Can you work these out from the model? Positions are in its coordinate system, mm. A direction names the side the tool comes from. Coordinates: 2 decimals unless noted, no trailing zeros. Loops run counter-clockwise (first coordinate to the right, second up) from the corner with the lowest first, then second, coordinate; pieces in that order, holes last.
Autodesk Inventor part; units mm, degrees
ref_plane "YZ Plane" through (0, 0, 0) normal (1, 0, 0) x (0, 1, 0)
ref_plane "XZ Plane" through (0, 0, 0) normal (0, 1, 0) x (-1, 0, 0)
ref_plane "XY Plane" through (0, 0, 0) normal (0, 0, 1) x (1, 0, 0)
sketch "Sketch1" plane through (0, 0, 0) normal (1, 0, 0) x (0, 1, 0)
  line L0 (-25.4, -50.8) -> (25.4, -50.8)
  line L1 (25.4, -50.8) -> (25.4, 50.8)
  line L2 (25.4, 50.8) -> (-25.4, 50.8)
  line L3 (-25.4, 50.8) -> (25.4, -50.8) construction
  line L4 (-25.4, -50.8) -> (25.4, 50.8) construction
  arc A0 (-25.4, -25.654) -> (-25.4, 25.654) centre (-25.4, 0) ccw
  line L5 (-25.4, 50.8) -> (-25.4, 25.654)
  line L6 (-25.4, -25.654) -> (-25.4, -50.8)
  point P0 (0, 0)
  dimension "d0" = 101.6
  dimension "d1" = 50.8
  dimension "d2" = 51.308
  dimension "d6" = 50.8
  dimension "d7" = 50.8
extrude "Extrusion1" add sketch "Sketch1" along normal mid plane 12.7
sketch "Sketch3" plane through (6.35, 0, 0) normal (1, 0, 0) x (0, 0, -1)
  circle A0 centre (0, -25.4) radius 31.75 construction
  point P0 (0, 0)
  point P1 (0, 6.35)
  point P2 (0, 6.35)
  point P3 (-27.4963, -9.525)
  point P4 (-27.4963, -41.275)
  point P5 (0, -57.15)
  point P6 (27.4963, -41.275)
  point P7 (27.4963, -9.525)
  dimension "d17" = 360
hole "Hole2" at (6.35, 6.35, 0) at (6.35, -9.525, 27.4963) at (6.35, -41.275, 27.4963) at (6.35, -57.15, 0) at (6.35, -41.275, -27.4963) at (6.35, -9.525, -27.4963) direction (-1, 0, 0) diameter 3.81 end through all
sketch "Sketch4" plane through (-6.35, 25.4, 50.8) normal (0, 1, 0) x (1, 0, 0)
  line L0 (12.7, 0) -> (0, 0) construction
  line L1 (6.35, 0) -> (6.35, 101.6) construction
  line L2 (12.7, 101.6) -> (0, 101.6) construction
  point P0 (6.35, 50.8)
  point P1 (6.35, 12.7)
  point P2 (6.35, 88.9)
  dimension "d26" = 12.7
  dimension "d27" = 12.7
hole "Hole3" at (0, 25.4, 38.1) at (0, 25.4, -38.1) direction (0, -1, 0) diameter 6.7564 end through all
sketch "Sketch5" plane through (-6.35, 25.4, 50.8) normal (0, 1, 0) x (1, 0, 0)
  circle A0 centre (6.35, 88.9) radius 3.3782
  circle A1 centre (6.35, 88.9) radius 4.0132
  circle A2 centre (6.35, 12.7) radius 3.3782
  circle A3 centre (6.35, 12.7) radius 4.0132
  point P0 (6.35, 50.8)
  dimension "d35" = 8.0264
extrude "Extrusion2" cut sketch "Sketch5" against normal blind 12.7
properties part number "BottomOfSupportForAxel" material "PBT Plastic"
(1) I want a section at A-A on y = 6.35. Write out the boundary of the cut face in (x, z) (3 decimals), then the cut area to 3 significant figures.
Check values:
outline: (-6.35, -50.8) - (6.35, -50.8) - (6.35, -1.905) - (-6.35, -1.905) - close; (-6.35, 1.905) - (6.35, 1.905) - (6.35, 50.8) - (-6.35, 50.8) - close; hole circle Ø6.756 at (0, -38.1); hole circle Ø6.756 at (0, 38.1)
area: 1,170 mm2
(2) I want a section at C-C on x = 0. Write out the boundary of the cut face in (y, z) (3 decimals), then the cut area to 3 significant figures.
Check values:
outline: (-25.4, -50.8) - (25.4, -50.8) - (25.4, -42.113) - (12.7, -42.113) - (12.7, -41.478) - (-25.4, -41.478) - close; (-25.4, -34.722) - (12.7, -34.722) - (12.7, -34.087) - (25.4, -34.087) - (25.4, 34.087) - (12.7, 34.087) - (12.7, 34.722) - (-25.4, 34.722) - (-25.4, 25.654) arc R25.654 cw to (-25.4, -25.654) - close; (-25.4, 41.478) - (12.7, 41.478) - (12.7, 42.113) - (25.4, 42.113) - (25.4, 50.8) - (-25.4, 50.8) - close; hole circle Ø3.81 at (-9.525, -27.496); hole circle Ø3.81 at (-9.525, 27.496); hole circle Ø3.81 at (6.35, 0)
area: 3,370 mm2
(3) If we mould it in two halves opening along X, with no side actions, what happens to faces 3 (the cylindrical face through (-0.149, -6.617, -41.475)), 4 (the flat face through (6.35, 11, 1)), 5 (the cylindrical face through (-0.09, 8.21, 0.41))? For each: released by +X, released by -X, zero draft, split by the parting line, or undercut.
Check values:
face 3: undercut
face 4: released by +X
face 5: zero draft
(4) If I drill on probe 1 along Z at (x, y) = (0, -10.5); probe 2 along Z at (x, y) = (0, -9.5); probe 3 along Z at (x, y) = (0, 15.75), over which ranges is the centre line in solid material (lowest first)?
Check values:
probe 1: z = -50.8 to -41.48, -34.72 to -29.13, -25.86 to -20.88, 20.88 to 25.86, 29.13 to 34.72, 41.48 to 50.8
probe 2: z = -50.8 to -41.48, -34.72 to -29.4, -25.59 to -20.13, 20.13 to 25.59, 29.4 to 34.72, 41.48 to 50.8
probe 3: z = -50.8 to -42.11, -34.09 to 34.09, 42.11 to 50.8
(5) I want a section at B-B on z = 0. Write out the boundary of the cut face in (x, y) (3 decimals).
Check values:
outline: (-6.35, 0.254) - (6.35, 0.254) - (6.35, 4.445) - (-6.35, 4.445) - close; (-6.35, 8.255) - (6.35, 8.255) - (6.35, 25.4) - (-6.35, 25.4) - close
(6) I want a section at D-D on z = -38.1. Write out the boundary of the cut face in (x, y).
Check values:
outline: (-6.35, -25.4) - (-3.38, -25.4) - (-3.38, 12.7) - (-4.01, 12.7) - (-4.01, 25.4) - (-6.35, 25.4) - close; (3.38, -25.4) - (6.35, -25.4) - (6.35, 25.4) - (4.01, 25.4) - (4.01, 12.7) - (3.38, 12.7) - close
(7) Which directions (+Z, -Z, +X, -X, +Y, -Y) give clear straight access to the entire face, cutting with the end or side of a thin tool? Please do faces 1 (the flat face through (0, 0, 50.8)), 2 (the cylindrical face through (-3.185, 19.139, 40.542)).
Check values:
face 1: +Z, +X, -X, +Y, -Y
face 2: +Y
(8) I'm going to push flat-ended pins straight in: pin 1 (2.5 mm diameter, centred on y = 6.35, z = 0, fed in from -X); pin 2 (2.5 mm diameter, centred on x = 2, z = -39.5, fed in from +Y). Where does each tip first touch, or does it pass through?
Check values:
pin 1: passes through
pin 2: stops at y = 12.7
